```python
from build123d import *
from build123d import SkipClean  # not in build123d's __all__

# Parameters (mm, degrees)
F0_W     = 24.5
F0_H     = 80
F1_DEPTH = 9.5
F3_D     = 5
F3_DEPTH = 22
F3_TIP   = 1.5021515476
F5_D     = 7
F5_DEPTH = 22
F5_TIP   = 2.1030121666
F7_ANGLE = 180


with BuildPart() as f1:
    # F0 (on Front) → F1 (new body, symmetric)
    with BuildSketch(Plane.XZ):
        with Locations((12.25, 0)):
            Rectangle(F0_W, F0_H)
    extrude(amount=F1_DEPTH, both=True)

    # F3
    with Locations(Plane.XY.offset(40)):
        with Locations((17.5, 0)):
            Hole(F3_D / 2, depth=F3_DEPTH)
            with Locations((0, 0, -(F3_DEPTH + F3_TIP / 2))):  # 118° drill point
                Cone(0, F3_D / 2, F3_TIP, mode=Mode.SUBTRACT)

    # F5
    with Locations(Plane(origin=(0, 0, -40), x_dir=(1, 0, 0), z_dir=(0, 0, -1))):
        with Locations((15, 0)):
            Hole(F5_D / 2, depth=F5_DEPTH)
            with Locations((0, 0, -(F5_DEPTH + F5_TIP / 2))):  # 118° drill point
                Cone(0, F5_D / 2, F5_TIP, mode=Mode.SUBTRACT)

    # F6 (on Right) → F7 (revolve, cut)
    with BuildSketch(Plane.YZ):
        with BuildLine():
            Line((-9.5, 0), (9.5, 0))
            Line((9.5, 0), (9.5, 15))
            Line((9.5, 15), (0.5, 15))
            Line((0.5, 15), (0.5, 17.5))
            ThreePointArc((0.5, 17.5), (0.2071067812, 18.2071067812), (-0.5, 18.5))
            Line((-0.5, 18.5), (-2, 18.5))
            ThreePointArc((-2, 18.5), (-2.5, 18.3660254038), (-2.8660254038, 18))
            Line((-2.8660254038, 18), (-3.1547005384, 17.5))
            Line((-3.1547005384, 17.5), (-9.5, 17.5))
            Line((-9.5, 17.5), (-9.5, 0))
        make_face()
    revolve(axis=Axis((0, 0, 0), (0, 1, 0)), revolution_arc=F7_ANGLE, mode=Mode.SUBTRACT)

    # F8: F1 across plane


with BuildPart() as f1_1:
    add(f1.part, clean=False)
    with SkipClean():  # cleaning this boolean's faces spoils the solid; the shape is the same uncleaned
        add(f1.part.mirror(Plane.YZ), clean=False)


solid = f1_1.part
```
The listing builds one solid part. Answer for the finished solid, in the listing's coordinates (mm). A direction names the side the tool comes from. Round coordinates to 2 decimals unless told otherwise and drop trailing zeros. Loops run counter-clockwise (first coordinate to the right, second up) from the corner with the lowest first, then second, coordinate; pieces in that order, holes last. Notation, with made-up numbers: (34, 67) - (58, 67) arc R28 cw to (58, 90) - close; hole circle Ø6 at (-37, 73.25). An arc over 180 degrees is marked (long way). Use one line per item in the form item = value. Start each with the question number.
1. A tool of negligible diameter and unlimited length cuts with its end or side. For faces 4 (the face through (0, 0, 40)), 5 (the face through (-11.66, -1.05, -28.85)), 6 (the face through (20, 0, 29)), 7 (the face through (10.648, -6.372, -13.887)), 8 (the face through (24.5, 0, -1)), from which of +Z, -Z, +X, -X, +Y, -Y can it reach the whole face along a straight path? Write none if from no direction.
2. The part is cut by section C-C on y = -4.5. Determine the outline of the cut face in (x, z), then the cut area to 3 significant figures.
3. The part is cut by section D-D on z = -24. Determine the outline of the cut face in (x, y), then the cut area to 3 significant figures.
4. The part is cut by section A-A on z = 0. Determine the outline of the cut face in (x, y), then the cut area to 3 significant figures.
5. The part is cut by section B-B on z = 35. Determine the outline of the cut face in (x, y), then the cut area to 3 significant figures.
6. For a pull along Z with two mould halves and no side action, classify faces 1 (the face through (17.155, -0.264, 16.759)), 2 (the face through (-0.66, 4.937, -14.985)), 3 (the face through (0, 0, -40)) as pulls with the +Z half, pulls with the -Z half, needs draft (parallel to the pull), parting line crosses it, or undercut.
7. Given pin 1 Ø1.5 at (x, z) = (14.5, 6.5) entering from -Y; pin 2 Ø6.5 at (x, y) = (15, 0) entering from -Z; pin 3 Ø1 at (x, y) = (-18.5, 1.5) entering from +Z, each flat-ended and moving along its own axis, determine where each tip first touches the part or whether it passes through.
8. Consider line 1 (X direction, y = 0, z = 25.75); line 2 (X direction, y = 4.75, z = 0); line 3 (Y direction, x = 15, z = -25). Determine where each line is inside the solid, lowest interval first. Write a range as [from, to].
Geometry check:
q1.face_4 = +Z, +X, -X, +Y, -Y
q1.face_5 = -Z
q1.face_6 = +Z
q1.face_7 = -Y
q1.face_8 = +Z, -Z, +X, +Y, -Y
q2.outline = (-24.5, -40) - (24.5, -40) - (24.5, 40) - (-24.5, 40) - close; hole circle Ø35 at (0, 0)
q2.area = 2,960 mm^2
q3.outline = (-24.5, -9.5) - (24.5, -9.5) - (24.5, 9.5) - (-24.5, 9.5) - close; hole circle Ø7 at (-15, 0); hole circle Ø7 at (15, 0)
q3.area = 854 mm^2
q4.outline = (-24.5, -9.5) - (-17.5, -9.5) - (-17.5, -3.15) - (-18, -2.87) arc R1 cw to (-18.5, -2) - (-18.5, -0.5) arc R1 cw to (-17.5, 0.5) - (-15, 0.5) - (-15, 9.5) - (-24.5, 9.5) - close; (15, 0.5) - (17.5, 0.5) arc R1 cw to (18.5, -0.5) - (18.5, -2) arc R1 cw to (18, -2.87) - (17.5, -3.15) - (17.5, -9.5) - (24.5, -9.5) - (24.5, 9.5) - (15, 9.5) - close
q4.area = 305 mm^2
q5.outline = (-24.5, -9.5) - (24.5, -9.5) - (24.5, 9.5) - (-24.5, 9.5) - close; hole circle Ø5 at (-17.5, 0); hole circle Ø5 at (17.5, 0)
q5.area = 892 mm^2
q6.face_1 = pulls with the +Z half
q6.face_2 = undercut
q6.face_3 = pulls with the -Z half
q7.pin_1 = 0.5
q7.pin_2 = -17.85
q7.pin_3 = 17.88
q8.line_1 = [-24.5, -20], [-15, 15], [20, 24.5]
q8.line_2 = [-24.5, -15], [15, 24.5]
q8.line_3 = [-9.5, -3.5], [3.5, 9.5]
